The model under review builds one solid part; all positions refer to its coordinate system, in mm. A direction names the side the tool comes from. Coordinates: 2 decimals unless noted, no trailing zeros. Write each loop counter-clockwise with the first axis right and the second up, starting at its lowest first coordinate (ties: lowest second). Pieces come first, ordered by that corner, then holes. Notation, with made-up numbers: (78.25, 7.25) -> (90.25, 7.25) arc R14 ccw to (90.25, 21.25) -> close; hole circle Ø9 at (81, 80). An arc over 180 degrees is marked (long way). Put each result on its own line as item: value. Start each with the question number.
Autodesk Inventor part; units mm, degrees
ref_plane "YZ Plane" through (0, 0, 0) normal (1, 0, 0) x (0, 1, 0)
ref_plane "XZ Plane" through (0, 0, 0) normal (0, 1, 0) x (-1, 0, 0)
ref_plane "XY Plane" through (0, 0, 0) normal (0, 0, 1) x (1, 0, 0)
sketch "Sketch1" plane through (0, 0, 0) normal (0, 1, 0) x (-1, 0, 0)
  line L0 (-37, 22) -> (37, 22) construction
  line L1 (37, 22) -> (37, -22) construction
  line L2 (37, -22) -> (-37, -22) construction
  line L3 (-37, -22) -> (-37, 22) construction
  line L4 (-37, 22) -> (37, -22) construction
  line L5 (37, 22) -> (-37, -22) construction
  line L6 (-47, 32) -> (47, 32) construction
  line L7 (47, 32) -> (47, -32) construction
  line L8 (47, -32) -> (-47, -32) construction
  line L9 (-47, -32) -> (-47, 32) construction
  line L10 (-47, 32) -> (47, -32) construction
  line L11 (47, 32) -> (-47, -32) construction
  line L12 (31, 16) -> (43, 16)
  line L13 (43, 16) -> (43, 28)
  line L14 (43, 28) -> (31, 28)
  line L15 (31, 28) -> (31, 16)
  line L16 (31, 16) -> (43, 28) construction
  line L17 (43, 16) -> (31, 28) construction
  line L18 (47, 0) -> (-47, 0) construction
  line L19 (0, 32) -> (0, -32) construction
  line L20 (37, -22) -> (-37, 22) construction
  line L21 (47, -32) -> (-47, 32) construction
  line L22 (31, -16) -> (43, -16)
  line L23 (43, -16) -> (43, -28)
  line L24 (43, -28) -> (31, -28)
  line L25 (31, -28) -> (31, -16)
  line L26 (31, -16) -> (43, -28) construction
  line L27 (43, -16) -> (31, -28) construction
  line L28 (-31, 16) -> (-43, 16)
  line L29 (-43, 16) -> (-43, 28)
  line L30 (-43, 28) -> (-31, 28)
  line L31 (-31, 28) -> (-31, 16)
  line L32 (-31, -16) -> (-43, -16)
  line L33 (-31, -28) -> (-31, -16)
  line L34 (-43, -28) -> (-31, -28)
  line L35 (-43, -16) -> (-43, -28)
  line L36 (43, 28) -> (-43, 28)
  line L37 (-43, 28) -> (-43, -28)
  line L38 (-43, -28) -> (43, -28)
  line L39 (43, -28) -> (43, 28)
  point P0 (0, 0)
  dimension "d0" = 74
  dimension "d1" = 44
  dimension "d2" = 10
  dimension "d3" = 10
  dimension "d4" = 12
  dimension "d5" = 12
extrude "Extrusion1" add sketch "Sketch1" against normal blind 5
extrude "Extrusion2" add sketch "Sketch1" against normal blind 30 contours L15 L14 L13 L12 | L23 L24 L25 L22 | L31 L28 L29 L30 | L34 L35 L32 L33
hole "Hole2" at (-37, 0, 22) at (-37, 0, -22) at (37, 0, -22) at (37, 0, 22) direction (0, -1, 0) diameter 3.4 depth 8 tip angle 118 countersink diameter 6.3 countersink angle 90
sketch "Sketch4" plane through (0, -30, 0) normal (0, -1, 0) x (1, 0, 0)
  line L0 (31, 28) -> (-31, 28)
  line L1 (-43, 16) -> (-31, 16)
  line L2 (31, 28) -> (-31, 28)
  line L3 (-31, 28) -> (-31, 16)
  line L4 (-31, 16) -> (31, 16)
  line L5 (31, 16) -> (31, 28)
  line L6 (43, -28) -> (-43, -28)
  line L7 (-43, -16) -> (-31, -16)
  line L8 (31, -28) -> (-31, -28)
  line L9 (-31, -28) -> (-31, -16)
  line L10 (-31, -16) -> (31, -16)
  line L11 (31, -16) -> (31, -28)
  point P0 (0, 0)
extrude "Extrusion3" add sketch "Sketch4" against normal blind 10
properties part number "PCB_Housing_01"
1. Tool access review of faces 1 (the cylindrical face through (38.5, -4.8, -21.2)), 2 (the flat face through (31, -12, 22)), 3 (the flat face through (1, -30, 22)): name each direction out of +Z, -Z, +X, -X, +Y, -Y from which nothing blocks a thin tool from reaching the whole face with its end or side.
2. Consider section B-B on z = -17.5. State the section outline as (x, y) points.
3. Consider section A-A on y = -23. State the section outline as (x, z) points.
4. The part is to be moulded in two halves that separate along X. For faces 4 (the flat face through (-43, -4.8, -0.4)), 5 (the flat face through (1, 0, 0)), 6 (the flat face through (1, -5, 0)), say which applies: released by +X, released by -X, zero draft, split by the parting line, or undercut.
5. Consider section C-C on x = -13.5. State the section outline as (y, z) points.
6. Wall thickness on line 1 (Z direction, x = -37, y = -5.25); line 2 (Z direction, x = -37, y = -3.5); line 3 (Z direction, x = 35, y = -20): over which ranges is each line inside the solid? List them lowest first. Write a range as from..to.
7. Insertion check: P1, Ø4, axis at x = -37, z = -22, coming from the +Y side; P2, Ø4, axis at x = 18, z = 13, coming from the -Y side; P3, Ø2.5, axis at x = 37, z = 22, coming from the +Y side. Each pin has a flat end and moves straight along its axis. Give the tip position at first contact, or say it passes through.
Output values:
1. face 1: +Y
1. face 2: +Z, -Z
1. face 3: +Z, -Z, +X, -X, -Y
2. outline: (-43, -30) -> (43, -30) -> (43, 0) -> (-43, 0) -> close; hole (-31, -20) -> (31, -20) -> (31, -5) -> (-31, -5) -> close
3. outline: (-43, -28) -> (43, -28) -> (43, -16) -> (-43, -16) -> close; (-43, 16) -> (43, 16) -> (43, 28) -> (-43, 28) -> close
4. face 4: released by -X
4. face 5: zero draft
4. face 6: undercut
5. outline: (-30, -28) -> (-20, -28) -> (-20, -16) -> (-30, -16) -> close; (-30, 16) -> (-20, 16) -> (-20, 28) -> (-30, 28) -> close; (-5, -28) -> (0, -28) -> (0, 28) -> (-5, 28) -> close
6. line 1: z = -28..-23.7, -20.3..-16, 16..20.3, 23.7..28
6. line 2: z = -28..-23.7, -20.3..20.3, 23.7..28
6. line 3: z = -28..-16, 16..28
7. P1: stops at y = -1.15
7. P2: stops at y = -5
7. P3: stops at y = -8.27
